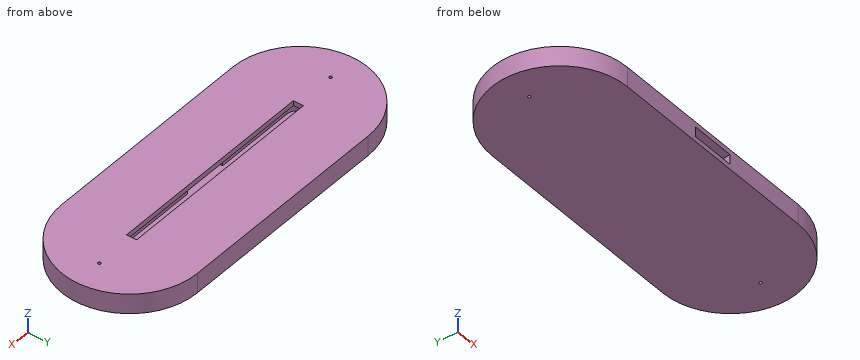
from build123d import *

# Parameters (mm, degrees)
PAD_DEPTH          = 9
POCKET_DEPTH       = 6
SKETCH002_W        = 26.5
SKETCH002_H        = 35
POCKET001_DEPTH    = 6
SKETCH003_W        = 127
SKETCH003_H        = 6
PAD001_DEPTH       = 3
SKETCH004_R        = 0.85
POCKET002_DEPTH    = 467.245989
POLARPATTERN_COUNT = 2


with BuildPart() as part:
    # Sketch → Pad (new body)
    with BuildSketch(Plane.XY):
        with BuildLine():
            ThreePointArc((-65, 41), (-106, 0), (-65, -41))
            Line((-65, -41), (65, -41))
            ThreePointArc((65, -41), (106, 0), (65, 41))
            Line((-65, 41), (65, 41))
        make_face()
    extrude(amount=PAD_DEPTH)

    # Sketch001 (on Face6 of Pad) → Pocket (cut)
    with BuildSketch(Plane.XY.offset(9)):
        with BuildLine():
            ThreePointArc((-62.5, 6), (-68.5, 0), (-62.5, -6))
            Line((-62.5, -6), (62.5, -6))
            ThreePointArc((62.5, -6), (68.5, 0), (62.5, 6))
            Line((-62.5, 6), (62.5, 6))
        make_face()
    extrude(amount=-POCKET_DEPTH, mode=Mode.SUBTRACT)

    # Sketch002 (on Face5 of Pocket) → Pocket001 (cut)
    with BuildSketch(Plane.XY.offset(9)):
        with Locations((0, -23.5)):
            Rectangle(SKETCH002_W, SKETCH002_H)
    extrude(amount=-POCKET001_DEPTH, mode=Mode.SUBTRACT)

    # Sketch003 (on Face5 of Pocket001) → Pad001 (join)
    with BuildSketch(Plane.XY.offset(9)):
        with BuildLine():
            ThreePointArc((-65, 41), (-106, 0), (-65, -41))
            Line((-65, -41), (65, -41))
            ThreePointArc((65, -41), (106, 0), (65, 41))
            Line((-65, 41), (65, 41))
        make_face()
        Rectangle(SKETCH003_W, SKETCH003_H, mode=Mode.SUBTRACT)
    extrude(amount=PAD001_DEPTH)

    # Sketch004 (on Face12 of Pad001) → Pocket002 (cut, through all)
    with BuildSketch(Plane.XY.offset(12)):
        with Locations((-88, 0)):
            Circle(SKETCH004_R)
    pocket002 = extrude(amount=-POCKET002_DEPTH, mode=Mode.SUBTRACT)

    # PolarPattern: Pocket002 ×2 about axis
    polarpattern_axis = Axis((0, 0, 12), (0, 0, 1))
    for i in range(1, POLARPATTERN_COUNT):
        add(pocket002.rotate(polarpattern_axis, i * 360 / POLARPATTERN_COUNT), mode=Mode.SUBTRACT)


solid = part.part
The listing builds one solid part. Answer for the finished solid, in the listing's coordinates (mm). Give positions to 0.01 mm unless a question says otherwise; leave off trailing zeros. Write each loop counter-clockwise with the first axis right and the second up, starting at its lowest first coordinate (ties: lowest second). Pieces come first, ordered by that corner, then holes. Notation, with made-up numbers: (9, 61) -> (16, 61) arc R12 cw to (16, 78) -> close; hole circle Ø1 at (0, 0.25). An arc over 180 degrees is marked (long way). One line per question, with ' | ' between items. Start each with the question number.
1. Section B-B (x = -18) is taken. Determine the outline of the cut face in (y, z).
2. Section A-A (x = 10) is taken. Determine the outline of the cut face in (y, z).
3. Find the intervals of material crossed by probe 1 along Z at (x, y) = (6, -22); probe 2 along Y at (x, z) = (-52.5, 4.75); probe 3 along Y at (x, z) = (-88, 8.5), in increasing order.
4. Section C-C (y = -31.5) is taken. Determine the outline of the cut face in (x, z), plus the area to 3 significant figures.
5. Section D-D (y = 32.5) is taken. Determine the outline of the cut face in (x, z) (3 decimals), plus the area to 3 significant figures.
6. Given pin 1 Ø0.9 at (y, z) = (0, 10.5) entering from +X; pin 2 Ø6.5 at (y, z) = (-24.5, 4.5) entering from +X; pin 3 Ø2 at (y, z) = (-12, 3.5) entering from +X, each flat-ended and moving along its own axis, determine where each tip first touches the part or whether it passes through.
Response values:
1) outline: (-41, 0) -> (41, 0) -> (41, 12) -> (3, 12) -> (3, 9) -> (6, 9) -> (6, 3) -> (-6, 3) -> (-6, 9) -> (-3, 9) -> (-3, 12) -> (-41, 12) -> close
2) outline: (-41, 0) -> (41, 0) -> (41, 12) -> (3, 12) -> (3, 9) -> (6, 9) -> (6, 3) -> (-41, 3) -> close; (-41, 9) -> (-3, 9) -> (-3, 12) -> (-41, 12) -> close
3) probe 1: 0 to 3, 9 to 12 | probe 2: -41 to -6, 6 to 41 | probe 3: -33.94 to -0.85, 0.85 to 33.94
4) outline: (-91.24, 0) -> (91.24, 0) -> (91.24, 12) -> (-91.24, 12) -> close; hole (-13.25, 3) -> (13.25, 3) -> (13.25, 9) -> (-13.25, 9) -> close | area: 2,030 mm2
5) outline: (-89.995, 0) -> (89.995, 0) -> (89.995, 12) -> (-89.995, 12) -> close | area: 2,160 mm2
6) pin 1: x = 106 | pin 2: x = 100.06 | pin 3: x = 104.5
